Part model, mm, in its own coordinate system. Coordinates: 2 decimals unless noted, no trailing zeros. Loops run counter-clockwise (first coordinate to the right, second up) from the corner with the lowest first, then second, coordinate; pieces in that order, holes last. Notation, with made-up numbers: (87.5, 54.25) - (116.5, 54.25) arc R34 cw to (116.5, 84.25) - close; hole circle Ø9 at (86.25, 23.5). An arc over 180 degrees is marked (long way). Use a Markdown table: item, result. Add a question column.
1) Probe probe 1 along X at (y, z) = (-190.5, 810); probe 2 along X at (y, z) = (-409, 203); probe 3 along X at (y, z) = (-608, 584). List the from-to ranges inside material, lowest first. Write a range as [from, to].
2) Band-saw the part on A-A (z = 349). Give the number of separate pieces and of enclosed holes in the cut face, plus the area to 3 significant figures.
3) Band-saw the part on D-D (y = -722.5). Give the cut face in (x, z).
4) Band-saw the part on B-B (y = -210). Give the cut face in (x, z).
5) Band-saw the part on C-C (x = 665). Give the cut face in (y, z), plus the area to 3 significant figures.
6) Drop a flat-ended pin along its axis: P1, Ø1, axis at x = 930.5, y = -535.5, coming from the -Z side. Give the stop position or say it passes through.
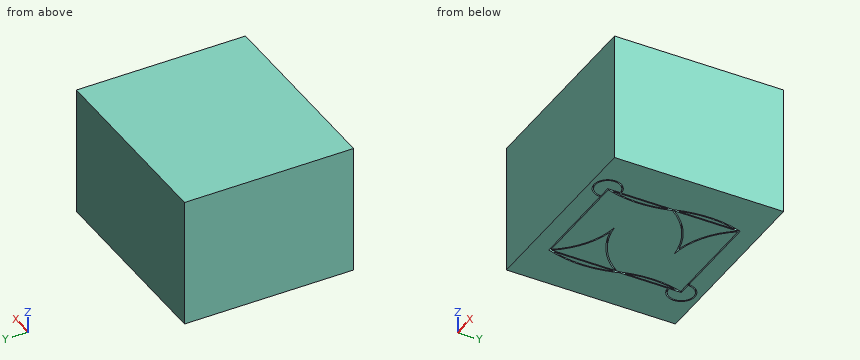
from build123d import *

# Parameters (mm, degrees)
SKETCH1_W                = 1500
SKETCH1_H                = 1300
BOSS_EXTRUDE3_DEPTH      = 1000
SKETCH5_W                = 820
SKETCH5_H                = 1020
SKETCH5_W_2              = 800
SKETCH5_H_2              = 1000
CUT_EXTRUDE_THIN5_DEPTH  = 900
CUT_EXTRUDE_THIN9_START  = -900
CUT_EXTRUDE_THIN9_DEPTH  = 900
CUT_EXTRUDE_THIN25_DEPTH = 900
CUT_EXTRUDE_THIN26_DEPTH = 900


# Read off the part's stored shape, not the designer's step: Cut-Extrude-Thin9
with BuildPart() as part:
    # Sketch1 → Boss-Extrude3 (new body)
    with BuildSketch(Plane(origin=(-226.705899875, 34.53488644, 0), x_dir=(1, 0, 0), z_dir=(0, 0, 1))):
        with Locations((666.978508717, -609.518449502)):
            Rectangle(SKETCH1_W, SKETCH1_H)
    extrude(amount=BOSS_EXTRUDE3_DEPTH)

    # Sketch5 → Cut-Extrude-Thin5 (cut)
    with BuildSketch(Plane(origin=(0, 0, 0), x_dir=(-1, 0, 0), z_dir=(0, 0, -1))):
        with Locations((-440.09863574, -578.647805533)):
            Rectangle(SKETCH5_W, SKETCH5_H)
        with Locations((-440.09863574, -578.647805533)):
            Rectangle(SKETCH5_W_2, SKETCH5_H_2, mode=Mode.SUBTRACT)
    extrude(amount=-CUT_EXTRUDE_THIN5_DEPTH, mode=Mode.SUBTRACT)

    # Cut-Extrude-Thin9 outline → Cut-Extrude-Thin9 (cut)
    with BuildSketch(Plane(origin=(0, 0, 0), x_dir=(-1, 0, 0), z_dir=(0, 0, -1)).offset(CUT_EXTRUDE_THIN9_START)):
        with BuildLine():
            ThreePointArc((-840.09863574, -612.777474084), (-810.032843418, -828.647805533), (-840.09863574, -1044.518136982))
            Line((-840.09863574, -1044.518136982), (-840.09863574, -1078.647805533))
            ThreePointArc((-840.09863574, -1078.647805533), (-800.032843418, -828.647805533), (-840.09863574, -578.647805533))
            Line((-840.09863574, -578.647805533), (-840.09863574, -612.777474084))
        make_face()
        with BuildLine():
            ThreePointArc((-40.09863574, -511.526312309), (-65.332815003, -313.452489118), (-40.09863574, -115.378665927))
            Line((-40.09863574, -115.378665927), (-40.09863574, -78.647805533))
            ThreePointArc((-40.09863574, -78.647805533), (-75.332815003, -313.452489118), (-40.09863574, -548.257172703))
            Line((-40.09863574, -548.257172703), (-40.09863574, -511.526312309))
        make_face()
        with BuildLine():
            ThreePointArc((-20.598154948, -575.520367878), (-25.486318472, -561.181617873), (-30.09863574, -546.751772975))
            Line((-30.09863574, -546.751772975), (-30.09863574, -578.647805533))
            ThreePointArc((-30.09863574, -578.647805533), (5.135543524, -813.452489118), (-30.09863574, -1048.257172703))
            Line((-30.09863574, -1048.257172703), (-30.09863574, -1080.348048155))
            ThreePointArc((-30.09863574, -1080.348048155), (14.992145049, -828.693386929), (-20.598154948, -575.520367878))
        make_face()
        with BuildLine():
            Line((-850.09863574, -111.389167393), (-850.09863574, -77.050278028))
            ThreePointArc((-850.09863574, -77.050278028), (-890.164428061, -328.647805533), (-850.09863574, -580.245333038))
            Line((-850.09863574, -580.245333038), (-850.09863574, -545.906443673))
            ThreePointArc((-850.09863574, -545.906443673), (-880.164428061, -328.647805533), (-850.09863574, -111.389167393))
        make_face()
    extrude(amount=CUT_EXTRUDE_THIN9_DEPTH, mode=Mode.SUBTRACT)

    # Sketch8 → Cut-Extrude-Thin25 (cut)
    with BuildSketch(Plane(origin=(0, 0, 0), x_dir=(-1, 0, 0), z_dir=(0, 0, -1))):
        with BuildLine():
            ThreePointArc((-44.204558678, -575.794492227), (-232.775541237, -750.064076456), (-477.220833635, -828.647805533))
            ThreePointArc((-477.220833635, -828.647805533), (-232.775541237, -907.231534609), (-44.204558678, -1081.501118839))
            Line((-44.204558678, -1081.501118839), (-35.992712801, -1075.794492227))
            ThreePointArc((-35.992712801, -1075.794492227), (-199.246048012, -916.307353384), (-409.967671451, -828.647805533))
            ThreePointArc((-409.967671451, -828.647805533), (-199.246048012, -740.988257682), (-35.992712801, -581.501118839))
            Line((-35.992712801, -581.501118839), (-44.204558678, -575.794492227))
        make_face()
        with BuildLine():
            ThreePointArc((-844.201980979, -81.504824582), (-680.110140526, -241.301950512), (-468.374562106, -328.647805533))
            ThreePointArc((-468.374562106, -328.647805533), (-680.110140526, -415.993660554), (-844.201980979, -575.790786484))
            Line((-844.201980979, -575.790786484), (-835.9952905, -581.504824582))
            ThreePointArc((-835.9952905, -581.504824582), (-645.344725951, -406.290174443), (-398.323524561, -328.647805533))
            ThreePointArc((-398.323524561, -328.647805533), (-645.344725951, -251.005436622), (-835.9952905, -75.790786484))
            Line((-835.9952905, -75.790786484), (-844.201980979, -81.504824582))
        make_face()
    extrude(amount=-CUT_EXTRUDE_THIN25_DEPTH, mode=Mode.SUBTRACT)

    # Sketch9 → Cut-Extrude-Thin26 (cut)
    with BuildSketch(Plane(origin=(0, 0, 0), x_dir=(-1, 0, 0), z_dir=(0, 0, -1))):
        with BuildLine():
            ThreePointArc((-30.09863574, -173.647805533), (44.147576285, 5.598406492), (-135.09863574, -68.647805533))
            Line((-135.09863574, -68.647805533), (-125.09863574, -68.647805533))
            ThreePointArc((-125.09863574, -68.647805533), (37.076508473, -1.47266132), (-30.09863574, -163.647805533))
            Line((-30.09863574, -163.647805533), (-30.09863574, -173.647805533))
        make_face()
        with BuildLine():
            ThreePointArc((-850.09863574, -983.647805533), (-924.344847764, -1162.894017558), (-745.09863574, -1088.647805533))
            Line((-745.09863574, -1088.647805533), (-755.09863574, -1088.647805533))
            ThreePointArc((-755.09863574, -1088.647805533), (-917.273779952, -1155.822949746), (-850.09863574, -993.647805533))
            Line((-850.09863574, -993.647805533), (-850.09863574, -983.647805533))
        make_face()
    extrude(amount=-CUT_EXTRUDE_THIN26_DEPTH, mode=Mode.SUBTRACT)


solid = part.part
Answer block:
| question | item | result |
|---|---|---|
| 1 | probe 1 | [-309.73, 30.1], [40.1, 55.71], [65.83, 731.47], [746.79, 840.1], [850.1, 868.15], [878.3, 1190.27] |
| 1 | probe 2 | [-309.73, 30.1], [40.1, 59.53], [69.61, 649.99], [669.22, 840.1], [850.1, 876.12], [886.17, 1190.27] |
| 1 | probe 3 | [-309.73, 11.35], [21.7, 30.1], [40.1, 55.5], [68.24, 831.06], [850.1, 1190.27] |
| 2 | separate pieces | 10 |
| 2 | enclosed holes | 1 |
| 2 | area | 1,870,000 mm2 |
| 3 | outline | (-309.73, 0) - (-10.01, 0) - (-10.01, 900) - (0.05, 900) - (0.05, 0) - (30.1, 0) - (30.1, 900) - (40.1, 900) - (40.1, 0) - (172.83, 0) - (172.83, 900) - (189.9, 900) - (189.9, 0) - (807.11, 0) - (807.11, 900) - (817.2, 900) - (817.2, 0) - (840.1, 0) - (840.1, 900) - (850.1, 900) - (850.1, 0) - (1190.27, 0) - (1190.27, 1000) - (-309.73, 1000) - close |
| 4 | outline | (-309.73, 0) - (30.1, 0) - (30.1, 900) - (40.1, 900) - (40.1, 0) - (58.53, 0) - (58.53, 900) - (68.62, 900) - (68.62, 0) - (707.09, 0) - (707.09, 900) - (723.42, 900) - (723.42, 0) - (840.1, 0) - (840.1, 900) - (850.1, 900) - (850.1, 0) - (871.32, 0) - (871.32, 900) - (881.43, 900) - (881.43, 0) - (1190.27, 0) - (1190.27, 1000) - (-309.73, 1000) - close |
| 5 | outline | (-1224.98, 0) - (-1088.65, 0) - (-1088.65, 900) - (-1078.65, 900) - (-1078.65, 0) - (-418.16, 0) - (-418.16, 900) - (-406.37, 900) - (-406.37, 0) - (-250.92, 0) - (-250.92, 900) - (-239.14, 900) - (-239.14, 0) - (-78.65, 0) - (-78.65, 900) - (-68.65, 900) - (-68.65, 0) - (75.02, 0) - (75.02, 1000) - (-1224.98, 1000) - close |
| 5 | area | 1,260,000 mm2 |
| 6 | P1 | z = 0 |
